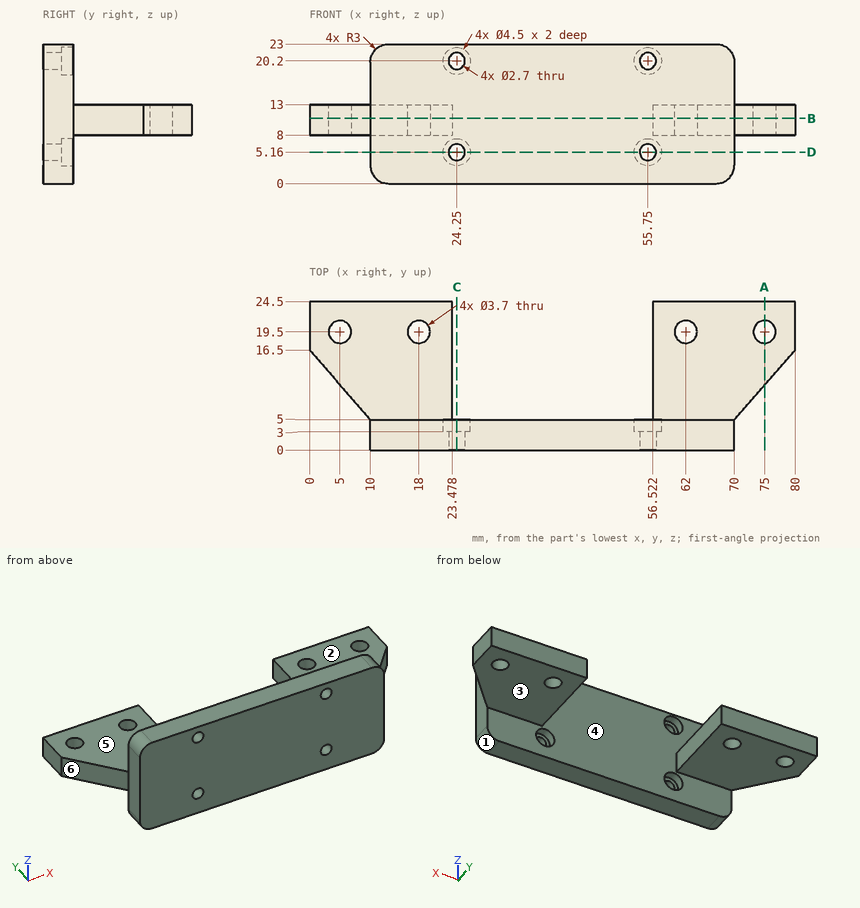
Geometry check sheet. Reference: drawing and pictorial views, mm from the part's lowest x, y, z. A direction names the side the tool comes from. Round coordinates to 2 decimals unless told otherwise and drop trailing zeros. Loops run counter-clockwise (first coordinate to the right, second up) from the corner with the lowest first, then second, coordinate; pieces in that order, holes last. Notation, with made-up numbers: (87.25, 24.5) - (125.25, 24.5) arc R11 ccw to (125.25, 40.5) - close; hole circle Ø9 at (28, -7). An arc over 180 degrees is marked (long way). Use a Markdown table: item, result. Add a question column.
1. Section check B-B, the plane z = 10.75. Record the boundary of the cut face in (x, y).
2. Section check C-C, the plane x = 24.25. Record the boundary of the cut face in (y, z), plus the area to 3 significant figures.
3. Access from +Z, -Z, +X, -X, +Y, -Y to the whole of each face (thin tool, end or side, straight path). Record for the marked faces 1, 2 and 3.
4. Thickness scan on probe 1 along X at (y, z) = (4.15, 20.2); probe 2 along X at (y, z) = (0.95, 20.2); probe 3 along X at (y, z) = (16.5, 12.5). Record the ranges inside material, lowest first. Write a range as [from, to].
5. Section check D-D, the plane z = 5.16. Record the boundary of the cut face in (x, y).
6. Gauge pin test, flat ends, axial feed: pin 1 (3 mm diameter, centred on x = 41.5, z = 4.5, fed in from -Y); pin 2 (5 mm diameter, centred on x = 23.5, z = 20, fed in from +Y); pin 3 (12 mm diameter, centred on y = 7, z = 18, fed in from +X) (1 decimal); pin 4 (5 mm diameter, centred on y = 5, z = 19, fed in from +X). Record the tip position at first contact, or that the pin passes through.
7. Release check for a two-part mould opening along X. For the marked faces 4, 5 and 6 record: released by +X, released by -X, zero draft, split by the parting line, or undercut.
8. Section check A-A, the plane x = 75. Record the boundary of the cut face in (y, z).
Checks:
| question | item | result |
|---|---|---|
| 1 | outline | (0, 16.5) - (10, 5) - (10, 0) - (70, 0) - (70, 5) - (80, 16.5) - (80, 24.5) - (56.52, 24.5) - (56.52, 5) - (23.48, 5) - (23.48, 24.5) - (0, 24.5) - close; hole circle Ø3.7 at (5, 19.5); hole circle Ø3.7 at (18, 19.5); hole circle Ø3.7 at (62, 19.5); hole circle Ø3.7 at (75, 19.5) |
| 2 | outline | (0, 0) - (5, 0) - (5, 2.91) - (3, 2.91) - (3, 3.81) - (0, 3.81) - close; (0, 6.51) - (3, 6.51) - (3, 7.41) - (5, 7.41) - (5, 17.95) - (3, 17.95) - (3, 18.85) - (0, 18.85) - close; (0, 21.55) - (3, 21.55) - (3, 22.45) - (5, 22.45) - (5, 23) - (0, 23) - close |
| 2 | area | 80.8 mm^2 |
| 3 | face 1 | -Z, +X, +Y, -Y |
| 3 | face 2 | +Z, +X, -X, +Y |
| 3 | face 3 | -Z, +X, -X, +Y |
| 4 | probe 1 | x = [10.01, 22], [26.5, 53.5], [58, 69.99] |
| 4 | probe 2 | x = [10.01, 22.9], [25.6, 54.4], [57.1, 69.99] |
| 4 | probe 3 | x = [0, 23.48], [56.52, 80] |
| 5 | outline | (10, 0) - (22.9, 0) - (22.9, 3) - (22, 3) - (22, 5) - (10, 5) - close; (25.6, 0) - (54.4, 0) - (54.4, 3) - (53.5, 3) - (53.5, 5) - (26.5, 5) - (26.5, 3) - (25.6, 3) - close; (57.1, 0) - (70, 0) - (70, 5) - (58, 5) - (58, 3) - (57.1, 3) - close |
| 6 | pin 1 | stops at y = 0 |
| 6 | pin 2 | stops at y = 5 |
| 6 | pin 3 | stops at x = 74.6 |
| 6 | pin 4 | stops at x = 70 |
| 7 | face 4 | undercut |
| 7 | face 5 | zero draft |
| 7 | face 6 | released by -X |
| 8 | outline | (10.75, 8) - (17.65, 8) - (17.65, 13) - (10.75, 13) - close; (21.35, 8) - (24.5, 8) - (24.5, 13) - (21.35, 13) - close |
